Model file for the job. Use its own axes, mm. Face numbers are marked on the shaded views. A direction names the side the tool comes from. Give positions to 0.01 mm unless a question says otherwise; leave off trailing zeros. Loops run counter-clockwise (first coordinate to the right, second up) from the corner with the lowest first, then second, coordinate; pieces in that order, holes last. Notation, with made-up numbers: M 2.5,27 L 56.5,27 A17 cw 56.5,50 Z; hole C -28,-21.5 d1. An arc over 180 degrees is marked long. Answer in a Markdown table with one row per item.
```python
from build123d import *

# Parameters (mm, degrees)
F0_R     = 22.86
F1_DEPTH = 25.4
F2_T     = -2.54
F3_R     = 2.9972
F4_DEPTH = 12.7
F5_R     = 9.964645
F6_DEPTH = 22.861


with BuildPart() as f1:
    # F0 (on Front) → F1 (new body)
    with BuildSketch(Plane.XZ):
        Circle(F0_R)
    extrude(amount=F1_DEPTH)

    # F2
    f2_openings = [f1.faces().sort_by_distance(p)[0] for p in [
        (0, -25.4, 0),
    ]]
    offset(amount=F2_T, openings=f2_openings)

    # F3 (on face) → F4 (cut, symmetric)
    with BuildSketch(Plane.XZ.offset(2.54)):
        Circle(F3_R)
    extrude(amount=F4_DEPTH, both=True, mode=Mode.SUBTRACT)

    # F5 (on Right) → F6 (cut, through all)
    with BuildSketch(Plane.YZ):
        with Locations((-12.170834, 0)):
            Circle(F5_R)
    extrude(amount=-F6_DEPTH, mode=Mode.SUBTRACT)


solid = f1.part
```
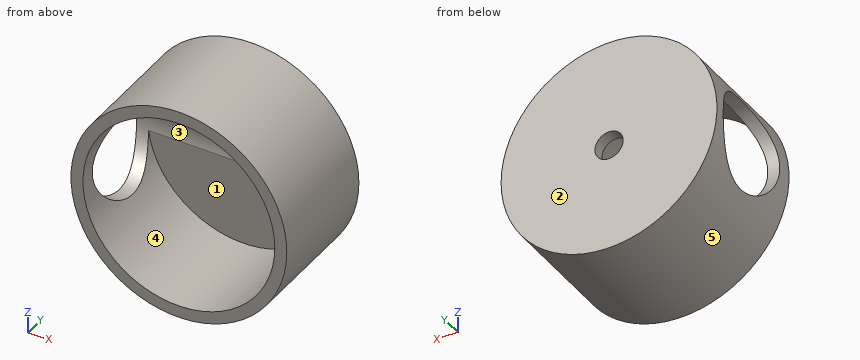
(1) Saw through at C-C, the plane x = 9. Give the cut face in (y, z), and give its area (3 significant figures).
Established:
| item | result |
|---|---|
| outline | M -25.4,-21.01 L 0,-21.01 L 0,21.01 L -25.4,21.01 L -25.4,18.22 L -2.54,18.22 L -2.54,-18.22 L -25.4,-18.22 Z |
| area | 235 mm2 |
(2) Wall check: L1, parallel to Z at x = 0, y = -12.5; L2, parallel to X at y = -1.45, z = 0; L3, parallel to Y at x = 18, z = -1. Give the ranges that are in metal, low to high.
Established:
| item | result |
|---|---|
| L1 | z = -22.86 to -20.32, 20.32 to 22.86 |
| L2 | x = -22.86 to -3, 3 to 22.86 |
| L3 | y = -2.54 to 0 |
(3) Mould opens along Y. For the marked faces 1, 2 and 3 say: pulls with the +Y half, pulls with the -Y half, needs draft (parallel to the pull), parting line crosses it, or undercut.
Established:
| item | result |
|---|---|
| face 1 | pulls with the -Y half |
| face 2 | pulls with the +Y half |
| face 3 | undercut |
(4) Flat gauge pins, fed straight in: P1, Ø4, axis at x = 13, z = 11.5, coming from the -Y side; P2, Ø10, axis at x = -16.5, y = -7, coming from the -Z side; P3, Ø2, axis at x = 6.5, y = -10, coming from the -Z side. Where does each tip first touch, or does it go through?
Established:
| item | result |
|---|---|
| P1 | stops at y = -2.54 |
| P2 | stops at z = -19.76 |
| P3 | stops at z = -22.19 |
(5) Saw through at B-B, the plane x = 0. Give the cut face in (y, z).
Established:
| item | result |
|---|---|
| outline | M -25.4,-22.86 L 0,-22.86 L 0,-3 L -2.54,-3 L -2.54,-20.32 L -25.4,-20.32 Z; M -25.4,20.32 L -2.54,20.32 L -2.54,3 L 0,3 L 0,22.86 L -25.4,22.86 Z |
(6) Saw through at A-A, the plane z = 0. Give the cut face in (x, y), and give its area (3 significant figures).
Established:
| item | result |
|---|---|
| outline | M -22.86,-25.4 L -20.32,-25.4 L -20.32,-22.14 L -22.86,-22.14 Z; M -22.86,-2.21 L -3,-2.21 L -3,0 L -22.86,0 Z; M 3,-2.54 L 20.32,-2.54 L 20.32,-25.4 L 22.86,-25.4 L 22.86,0 L 3,0 Z |
| area | 161 mm2 |
(7) Saw through at D-D, the plane z = 17.5. Give the cut face in (x, y).
Established:
| item | result |
|---|---|
| outline | M -14.71,-25.4 L -10.33,-25.4 L -10.33,-2.54 L 10.33,-2.54 L 10.33,-25.4 L 14.71,-25.4 L 14.71,0 L -14.71,0 Z |
(8) Which spindle directions (+Z, -Z, +X, -X, +Y, -Y) get a long thin tool onto all of the face, cutting with end or side? Do the marked faces 4 and 5. Say none if no direction does.
Established:
| item | result |
|---|---|
| face 4 | -Y |
| face 5 | +Y, -Y |
